Model file for the job. Use its own axes, mm. Face numbers are marked on the shaded views. A direction names the side the tool comes from. Coordinates: 2 decimals unless noted, no trailing zeros. Write each loop counter-clockwise with the first axis right and the second up, starting at its lowest first coordinate (ties: lowest second). Pieces come first, ordered by that corner, then holes.
Q1. Band-saw the part on A-A, the plane z = 0. Write the cut outline in (x, y), plus the area to 3 significant figures.
Q2. Band-saw the part on D-D, the plane y = 15.1. Write the cut outline in (x, z), plus the area to 3 significant figures.
Q3. Drill centre lines: probe 1 along X at (y, z) = (4, 0); probe 2 along X at (y, z) = (29.5, 10.5); probe 3 along Z at (x, y) = (-40, 6). Where is each one in solid material? Low to high.
Q4. Pin check, flat tips, straight feed: P1, Ø10, axis at x = -20.5, z = 4, coming from the +Y side; P2, Ø6, axis at x = -39.5, z = -11, coming from the +Y side; P3, Ø4, axis at y = 11.5, z = -11.5, coming from the +X side; P4, Ø4, axis at y = 20.5, z = -11.5, coming from the -X side. Stop position of each tip, or through.
Q5. Which spindle directions (+Z, -Z, +X, -X, +Y, -Y) get a long thin tool onto all of the face, cutting with end or side? Do the marked faces 4 and 5. Say none if no direction does.
Q6. Band-saw the part on B-B, the plane z = 16.5. Write the cut outline in (x, y).
Q7. Pull direction X, two halves, no side cores. Call the marked faces 1, 2 and 3: released by +X, released by -X, zero draft, split by the parting line, or undercut.
Q8. Band-saw the part on C-C, the plane y = 36.5. Write the cut outline in (x, z), plus the area to 3 significant figures.
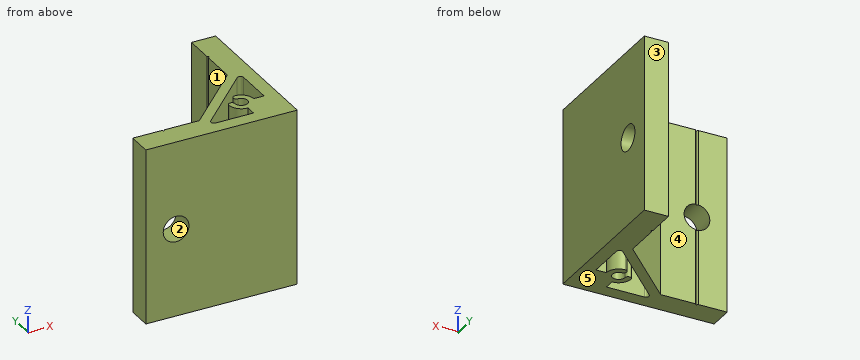
from build123d import *

# Parameters (mm, degrees)
EXTRUDE_1_DEPTH     = 29
SKETCH_2_R          = 4.25
CUT_EXTRUDE_1_DEPTH = 9
SKETCH_3_R          = 4.25
CUT_EXTRUDE_2_DEPTH = 9


with BuildPart() as part:
    # Эскиз1 → Бобышка-Вытянуть1 (new body, symmetric)
    with BuildSketch(Plane.XY):
        Polygon((-50, 0), (0, 0), (0, 50), (-8, 50), (-8, 40.5), (-7.5, 40), (-8, 39.5), (-8, 28), (-28, 8), (-39.5, 8), (-40, 7.5), (-40.5, 8), (-50, 8), align=None)
        with BuildLine():
            Line((-4.5, 12), (-4.5, 24.560303038))
            ThreePointArc((-4.5, 24.560303038), (-5.117316568, 25.484182571), (-6.207106781, 25.267409819))
            Line((-6.207106781, 25.267409819), (-25.267409819, 6.207106781))
            ThreePointArc((-25.267409819, 6.207106781), (-25.484182571, 5.117316568), (-24.560303038, 4.5))
            Line((-24.560303038, 4.5), (-12, 4.5))
            Line((-12, 4.5), (-12, 7.9))
            ThreePointArc((-12, 7.9), (-14.899137803, 9.100862197), (-16.1, 12))
            ThreePointArc((-16.1, 12), (-15.1, 13), (-14.1, 12))
            ThreePointArc((-14.1, 12), (-10.51507576, 10.51507576), (-12, 14.1))
            ThreePointArc((-12, 14.1), (-13, 15.1), (-12, 16.1))
            ThreePointArc((-12, 16.1), (-9.100862197, 14.899137803), (-7.9, 12))
            Line((-7.9, 12), (-4.5, 12))
        make_face(mode=Mode.SUBTRACT)
    extrude(amount=EXTRUDE_1_DEPTH, both=True)

    # Эскиз2 → Вырез-Вытянуть1 (cut, through all)
    with BuildSketch(Plane.ZY.offset(8)):
        with Locations(Location((0, 40, 0), (0, 0, 270))):  # turned: the seam where the file's is
            Circle(SKETCH_2_R)
    extrude(amount=-CUT_EXTRUDE_1_DEPTH, mode=Mode.SUBTRACT)

    # Эскиз3 → Вырез-Вытянуть2 (cut, through all)
    with BuildSketch(Plane(origin=(0, 8, 0), x_dir=(1, 0, 0), z_dir=(0, 1, 0))):
        with Locations(Location((-40, 0, 0), (0, 0, 180))):  # turned: the seam where the file's is
            Circle(SKETCH_3_R)
    extrude(amount=-CUT_EXTRUDE_2_DEPTH, mode=Mode.SUBTRACT)


solid = part.part
Answer sheet:
1. outline: (-50, 0) - (-44.25, 0) - (-44.25, 8) - (-50, 8) - close; (-35.75, 0) - (0, 0) - (0, 35.75) - (-8, 35.75) - (-8, 28) - (-28, 8) - (-35.75, 8) - close; (-8, 44.25) - (0, 44.25) - (0, 50) - (-8, 50) - close; hole (-25.27, 6.21) arc R1 ccw to (-24.56, 4.5) - (-12, 4.5) - (-12, 7.9) arc R4.1 cw to (-16.1, 12) arc R1 cw to (-14.1, 12) arc R2.1 ccw (long way) to (-12, 14.1) arc R1 cw to (-12, 16.1) arc R4.1 cw to (-7.9, 12) - (-4.5, 12) - (-4.5, 24.56) arc R1 ccw to (-6.21, 25.27) - close
1. area: 625 mm2
2. outline: (-20.9, -29) - (-16.37, -29) - (-16.37, 29) - (-20.9, 29) - close; (-13, -29) - (-9.32, -29) - (-9.32, 29) - (-13, 29) - close; (-4.5, -29) - (0, -29) - (0, 29) - (-4.5, 29) - close
2. area: 737 mm2
3. probe 1: x = -50 to -44.25, -35.75 to 0
3. probe 2: x = -8 to 0
3. probe 3: z = -29 to -4.25, 4.25 to 29
4. P1: stops at y = 20.5
4. P2: stops at y = 8
4. P3: stops at x = 0
4. P4: stops at x = -17.5
5. face 4: +Z, -Z, -X, +Y
5. face 5: -Z, +X, -X, +Y, -Y
6. outline: (-50, 0) - (0, 0) - (0, 50) - (-8, 50) - (-8, 40.5) - (-7.5, 40) - (-8, 39.5) - (-8, 28) - (-28, 8) - (-39.5, 8) - (-40, 7.5) - (-40.5, 8) - (-50, 8) - close; hole (-25.27, 6.21) arc R1 ccw to (-24.56, 4.5) - (-12, 4.5) - (-12, 7.9) arc R4.1 cw to (-16.1, 12) arc R1 cw to (-14.1, 12) arc R2.1 ccw (long way) to (-12, 14.1) arc R1 cw to (-12, 16.1) arc R4.1 cw to (-7.9, 12) - (-4.5, 12) - (-4.5, 24.56) arc R1 ccw to (-6.21, 25.27) - close
7. face 1: released by -X
7. face 2: undercut
7. face 3: zero draft
8. outline: (-8, -29) - (0, -29) - (0, -2.41) - (-8, -2.41) - close; (-8, 2.41) - (0, 2.41) - (0, 29) - (-8, 29) - close
8. area: 425 mm2
